from build123d import *

# Parameters (mm, degrees)
SKETCH1_W           = 20
SKETCH1_H           = 22.5
BOSS_EXTRUDE1_DEPTH = 30
SKETCH2_W           = 40
SKETCH2_H           = 40
BOSS_EXTRUDE2_DEPTH = 20
FILLET1_R           = 10


with BuildPart() as part:
    # Sketch1 → Boss-Extrude1 (new body)
    with BuildSketch(Plane.XY):
        with Locations((-20, -11.25)):
            Rectangle(SKETCH1_W, SKETCH1_H)
    extrude(amount=BOSS_EXTRUDE1_DEPTH)

    # Sketch2 → Boss-Extrude2 (add)
    with BuildSketch(Plane.XY):
        with Locations((-10, -2.5)):
            Rectangle(SKETCH2_W, SKETCH2_H)
    extrude(amount=-BOSS_EXTRUDE2_DEPTH)

    # Fillet1
    fillet1_edges = [part.edges().sort_by_distance(p)[0] for p in [
        (-20, 0, 0),
    ]]
    fillet(fillet1_edges, radius=FILLET1_R)
    fillet1_2_edges = [part.edges().sort_by_distance(p)[0] for p in [
        (10, 17.5, -10),
        (-20, 0, 30),
    ]]
    fillet(fillet1_2_edges, radius=FILLET1_R)


solid = part.part
Geometry: final body of the model. Coordinates: model frame, mm. A direction names the side the tool comes from. Round coordinates to 2 decimals unless told otherwise and drop trailing zeros. Order: outer loops, then holes, each group sorted by start corner. A loop starts at its lowest first (then second) coordinate and runs counter-clockwise, first axis right, second up. Notation, with made-up numbers: (-8.5, -38) - (29.5, -38) arc R28 ccw to (29.5, -3) - close; hole circle Ø9 at (-30, -26). An arc over 180 degrees is marked (long way). Write each question's results on one line, items separated by ' | '.
Item 1: Section A-A, the plane x = -14. Return the cut outline in (y, z), and give its area (4 significant figures).
Completed:
outline: (-22.5, -20) - (17.5, -20) - (17.5, 0) - (10, 0) arc R10 cw to (0, 10) - (0, 20) arc R10 ccw to (-10, 30) - (-22.5, 30) - close | area: 1,475 mm^2
Item 2: Section D-D, the plane y = -6. Return the cut outline in (x, z).
Completed:
outline: (-30, -20) - (10, -20) - (10, 0) - (-10, 0) - (-10, 29.17) - (-30, 29.17) - close
Item 3: Reachability of faces 1 (the flat face through (-10, -2, -20)), 2 (the flat face through (-6, 2, 0)), 3 (the flat face through (-10, -10, 15)), 4 (the flat face through (-20, 0, 15)), 5 (the flat face through (10, -8, -10)) from +Z, -Z, +X, -X, +Y, -Y: full face, straight path, thin tool, end or side. Return the list, or none.
Completed:
face 1: -Z, +X, -X, +Y, -Y | face 2: +Z, +X, +Y | face 3: +Z, +X, +Y, -Y | face 4: +Z, +X, -X, +Y | face 5: +Z, -Z, +X, +Y, -Y
Item 4: Material intervals for line 1 along Z through (x, y) = (-3, 13.5); line 2 along X through (y, z) = (-8.5, 12); line 3 along X through (y, z) = (9.5, -9), sorted ascending. Write a range as [from, to].
Completed:
line 1: [-20, 0] | line 2: [-30, -10] | line 3: [-30, 9.8]
Item 5: First-contact query: pin 1 Ø2 at (x, z) = (-12.5, 6.5) entering from +Y; pin 2 Ø11 at (x, z) = (-16, 15) entering from +Y; pin 3 Ø10 at (x, y) = (-14, 2) entering from +Z. Flat tips, straight axial feed; report the tip coordinate or a pass-through.
Completed:
pin 1: y = 1.07 | pin 2: y = 0.01 | pin 3: z = 27.14
Item 6: Section B-B, the plane y = -18. Return the cut outline in (x, z), and give its area (3 significant figures).
Completed:
outline: (-30, -20) - (10, -20) - (10, 0) - (-10, 0) - (-10, 30) - (-30, 30) - close | area: 1,400 mm^2
Item 7: Section C-C, the plane x = -3.5. Return the cut outline in (y, z).
Completed:
outline: (-22.5, -20) - (17.5, -20) - (17.5, 0) - (-22.5, 0) - close
